Check sheet for the modelled part. Datum: model origin and axes. Units: mm. A direction names the side the tool comes from. Round coordinates to 2 decimals unless told otherwise and drop trailing zeros. Write each loop counter-clockwise with the first axis right and the second up, starting at its lowest first coordinate (ties: lowest second). Pieces come first, ordered by that corner, then holes. Notation, with made-up numbers: (85, 69.25) - (114, 69.25) arc R21 ccw to (114, 94.25) - close; hole circle Ø11 at (82, -31). An arc over 180 degrees is marked (long way). Use one line per item in the form item = value. Start each with the question number.
1) Draft check along X on faces 1 (the face through (0, 27.5, 1)), 2 (the face through (-14, -8, 2)), 3 (the face through (-17.5, 0, 1)), 4 (the face through (13.4, -16.93, 1.48)). Enter one of: +X half, -X half, draft (parallel to the pull), parting line (faces both ways), or undercut.
2) Set-up check for faces 5 (the face through (15, 26, 1)), 6 (the face through (0, 2.5, 2)): record each of +Z, -Z, +X, -X, +Y, -Y from which the full face is reachable in a straight line by a thin tool's end or side.
3) Section check C-C (x = 0). Record the boundary of the cut face in (y, z), then the cut area to 3 significant figures.
4) Section check B-B (y = -3.5). Record the boundary of the cut face in (x, z), then the cut area to 3 significant figures.
5) Section check D-D (z = 2.35). Record the boundary of the cut face in (x, y).
6) Section check A-A (x = 8). Record the boundary of the cut face in (y, z).
7) Gauge pin test, flat end, axial feed: P1, Ø3, axis at x = 0, y = 23.5, coming from the +Z side. Record the tip position at first contact, or that the pin passes through.
8) Scan lines: probe 1 along Y at (x, z) = (0, 1.5); probe 2 along Y at (x, z) = (10.5, 2.85); probe 3 along Y at (x, z) = (-12.5, 0.8). Record each from-to range of solid material in increasing order.
from build123d import *

# Parameters (mm, degrees)
SKETCH_1_W                  = 35
SKETCH_1_H                  = 55
EXTRUDE_1_DEPTH             = 3
CHAMFER_1_SIZE              = 4
SKETCH_2_R                  = 1.6
CUT_EXTRUDE_1_DEPTH         = 33.733774607
PATTERN_LINEAR_1_COUNT      = 2
PATTERN_LINEAR_1_PITCH      = 25
PATTERN_LINEAR_1_COUNT_DIR2 = 2
PATTERN_LINEAR_1_PITCH_DIR2 = 30
SKETCH_3_R                  = 1.6
CUT_EXTRUDE_2_DEPTH         = 33.733774607
PATTERN_LINEAR_2_COUNT      = 2
PATTERN_LINEAR_2_PITCH      = 8
SKETCH_4_W                  = 28
SKETCH_4_H                  = 20
CUT_EXTRUDE_3_DEPTH         = 33.733774607
FILLET_1_R                  = 2


with BuildPart() as part:
    # 草圖1 → 填料-伸長1 (new body)
    with BuildSketch(Plane.XY):
        Rectangle(SKETCH_1_W, SKETCH_1_H)
    extrude(amount=EXTRUDE_1_DEPTH)

    # 導角1
    chamfer_1_edges = [part.edges().sort_by_distance(p)[0] for p in [
        (-17.5, 27.5, 1.5),
        (17.5, 27.5, 1.5),
        (17.5, -27.5, 1.5),
        (-17.5, -27.5, 1.5),
    ]]
    chamfer(chamfer_1_edges, length=CHAMFER_1_SIZE)

    # 草圖2 → 除料-伸長1 (cut, through all)
    with BuildSketch(Plane.XY.offset(3)):
        with Locations((-12.5, 7.5)):
            Circle(SKETCH_2_R)
    cut_extrude_1 = extrude(amount=-CUT_EXTRUDE_1_DEPTH, mode=Mode.SUBTRACT)

    # 直線複製排列1: Cut-Extrude 1 2 × 2
    with Locations(*[(i * PATTERN_LINEAR_1_PITCH, -j * PATTERN_LINEAR_1_PITCH_DIR2, 0) for i in range(PATTERN_LINEAR_1_COUNT) for j in range(PATTERN_LINEAR_1_COUNT_DIR2) if (i, j) != (0, 0)]):
        add(cut_extrude_1, mode=Mode.SUBTRACT)

    # 草圖3 → 除料-伸長2 (cut, through all)
    with BuildSketch(Plane.XY.offset(3)):
        with Locations((0, 23.5)):
            Circle(SKETCH_3_R)
    cut_extrude_2 = extrude(amount=-CUT_EXTRUDE_2_DEPTH, mode=Mode.SUBTRACT)

    # 直線複製排列2: 除料-伸長2 ×2
    with Locations(*[(0, -i * PATTERN_LINEAR_2_PITCH, 0) for i in range(1, PATTERN_LINEAR_2_COUNT)]):
        add(cut_extrude_2, mode=Mode.SUBTRACT)

    # 草圖4 → 除料-伸長3 (cut, through all)
    with BuildSketch(Plane.XY.offset(3)):
        with Locations((0, -7.5)):
            Rectangle(SKETCH_4_W, SKETCH_4_H)
    extrude(amount=-CUT_EXTRUDE_3_DEPTH, mode=Mode.SUBTRACT)

    # 圓角1
    fillet_1_edges = [part.edges().sort_by_distance(p)[0] for p in [
        (-14, -17.5, 1.5),
        (-14, 2.5, 1.5),
        (14, 2.5, 1.5),
        (14, -17.5, 1.5),
    ]]
    fillet(fillet_1_edges, radius=FILLET_1_R)


solid = part.part
Results are:
q1.face_1 = draft
q1.face_2 = undercut
q1.face_3 = -X half
q1.face_4 = undercut
q2.face_5 = +Z, -Z, +X, +Y
q2.face_6 = +Z, -Z
q3.outline = (-27.5, 0) - (-17.5, 0) - (-17.5, 3) - (-27.5, 3) - close; (2.5, 0) - (13.9, 0) - (13.9, 3) - (2.5, 3) - close; (17.1, 0) - (21.9, 0) - (21.9, 3) - (17.1, 3) - close; (25.1, 0) - (27.5, 0) - (27.5, 3) - (25.1, 3) - close
q3.area = 85.8 mm²
q4.outline = (-17.5, 0) - (-14, 0) - (-14, 3) - (-17.5, 3) - close; (14, 0) - (17.5, 0) - (17.5, 3) - (14, 3) - close
q4.area = 21.0 mm²
q5.outline = (-17.5, -23.5) - (-13.5, -27.5) - (13.5, -27.5) - (17.5, -23.5) - (17.5, 23.5) - (13.5, 27.5) - (-13.5, 27.5) - (-17.5, 23.5) - close; hole circle Ø3.2 at (-12.5, -22.5); hole circle Ø3.2 at (-12.5, 7.5); hole (-14, -15.5) arc R2 ccw to (-12, -17.5) - (12, -17.5) arc R2 ccw to (14, -15.5) - (14, 0.5) arc R2 ccw to (12, 2.5) - (-12, 2.5) arc R2 ccw to (-14, 0.5) - close; hole circle Ø3.2 at (0, 15.5); hole circle Ø3.2 at (0, 23.5); hole circle Ø3.2 at (12.5, -22.5); hole circle Ø3.2 at (12.5, 7.5)
q6.outline = (-27.5, 0) - (-17.5, 0) - (-17.5, 3) - (-27.5, 3) - close; (2.5, 0) - (27.5, 0) - (27.5, 3) - (2.5, 3) - close
q7.P1 = through
q8.probe_1 = -27.5 to -17.5, 2.5 to 13.9, 17.1 to 21.9, 25.1 to 27.5
q8.probe_2 = -27.5 to -17.5, 2.5 to 27.5
q8.probe_3 = -27.5 to -24.1, -20.9 to -17.44, 2.44 to 5.9, 9.1 to 27.5
